Design review of the part built by this model. Coordinates are the model's own, in mm. Face numbers are marked on the shaded views. Coordinates: 2 decimals unless noted, no trailing zeros. Order: outer loops, then holes, each group sorted by start corner. A loop starts at its lowest first (then second) coordinate and runs counter-clockwise, first axis right, second up.
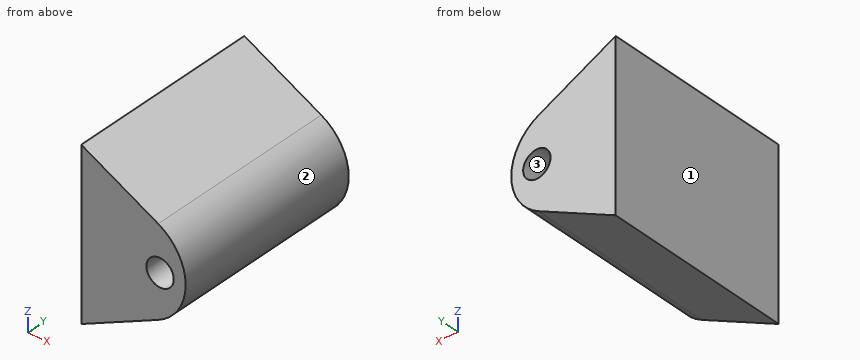
from build123d import *

# Parameters (mm, degrees)
BOSS_EXTRUDE1_DEPTH         = 23
FILLET1_R                   = 6
PREFORO_DA_MASCHIARE_M4_1_D = 3.3
BODY_MOVE_COPY1_ANGLE       = 90


with BuildPart() as part:
    # Sketch2 → Boss-Extrude1 (new body)
    with BuildSketch(Plane(origin=(0, 0, 0), x_dir=(0, 0, -1), z_dir=(1, 0, 0))):
        Polygon((-58.658771552, 3.364610889), (-38.658771552, 3.364610889), (-48.658771552, -16.635389111), align=None)
    extrude(amount=BOSS_EXTRUDE1_DEPTH)

    # Fillet1
    fillet1_edges = [part.edges().sort_by_distance(p)[0] for p in [
        (11.5, -16.635389111, 48.658771552),
    ]]
    fillet(fillet1_edges, radius=FILLET1_R)

    # Preforo da maschiare M4-1 (through all)
    with Locations(Plane.ZY):
        with Locations((48.658771552, -6.135389111)):
            Hole(PREFORO_DA_MASCHIARE_M4_1_D / 2)


with BuildPart() as part_1:
    # Body-Move/Copy1: moved
    add(part.part.rotate(Axis((10, -2.927185179, 0), (0, 0, 1)), BODY_MOVE_COPY1_ANGLE))


solid = part_1.part
1. Add section B-B (y = -8). Give the boundary of the cut face in (x, z).
2. Add section C-C (z = 44.75). Give the boundary of the cut face in (x, y), and give its area (3 significant figures).
3. Mouldability with a two-part tool opening along X and no side actions: class the marked faces 1, 2 and 3 as pulls with the +X half, pulls with the -X half, needs draft (parallel to the pull), parting line crosses it, or undercut.
4. Insertion check: pin 1 (12 mm diameter, centred on y = -1.5, z = 55, fed in from +X); pin 2 (2 mm diameter, centred on x = 13.5, y = 1, fed in from +Z); pin 3 (5 mm diameter, centred on x = 7, y = 3, fed in from -Z). Each pin has a flat end and moves straight along its axis. Give the tip position at first contact, or say it passes through.
5. To check wall thickness, follow line 1 (Z direction, x = 13.25, y = -10.5); line 2 (Z direction, x = 15, y = 4.5); line 3 (Z direction, x = 5, y = 4.25). State the ranges of each line that lie inside material, in increasing order.
6. Add section D-D (x = 8.5). Give the boundary of the cut face in (y, z), and give its area (3 significant figures).
7. Add section A-A (x = 12). Give the boundary of the cut face in (y, z), and give its area (3 significant figures).
Solution:
1. outline: (3.71, 38.66) - (12.98, 43.29) arc R6 ccw to (12.98, 54.03) - (3.71, 58.66) - close; hole circle Ø3.3 at (13.21, 48.66)
2. outline: (3.71, -12.93) - (14.84, -12.93) - (14.84, 10.07) - (3.71, 10.07) - close
2. area: 256 mm2
3. face 1: pulls with the -X half
3. face 2: pulls with the +X half
3. face 3: undercut
4. pin 1: stops at x = 16.28
4. pin 2: stops at z = 54.26
4. pin 3: stops at z = 39.05
5. line 1: z = 43.44 to 47.01, 50.31 to 53.88
5. line 2: z = 44.94 to 52.38
5. line 3: z = 39.3 to 58.01
6. outline: (-12.93, 41.05) - (10.07, 41.05) - (10.07, 56.26) - (-12.93, 56.26) - close
6. area: 350 mm2
7. outline: (-12.93, 42.8) - (10.07, 42.8) - (10.07, 47.54) - (-12.93, 47.54) - close; (-12.93, 49.78) - (10.07, 49.78) - (10.07, 54.51) - (-12.93, 54.51) - close
7. area: 218 mm2
